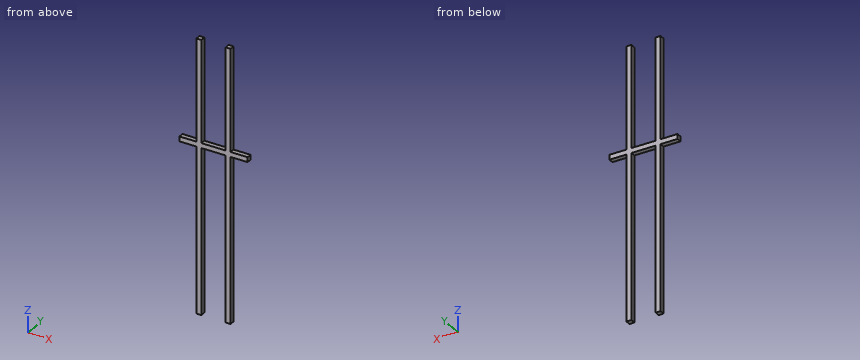
```python
from build123d import *

# Parameters (mm, degrees)
F1_DEPTH = 25.4


with BuildPart() as f1:
    # F0 (on Front) → F1 (new body)
    with BuildSketch(Plane.XZ):
        Polygon((-63.5, 546.1), (-88.9, 546.1), (-88.9, 12.7), (-177.8, 12.7), (-177.8, -12.7), (-88.9, -12.7), (-88.9, -876.3), (-63.5, -876.3), (-63.5, -12.7), (63.5, -12.7), (63.5, -876.3), (88.9, -876.3), (88.9, -12.7), (177.8, -12.7), (177.8, 12.7), (88.9, 12.7), (88.9, 546.1), (63.5, 546.1), (63.5, 12.7), (-63.5, 12.7), align=None)
    extrude(amount=-F1_DEPTH)


solid = f1.part
```
Work out the finished part from the listing and answer in its coordinate system (mm). Give positions to 0.01 mm unless a question says otherwise; leave off trailing zeros. Write each loop counter-clockwise with the first axis right and the second up, starting at its lowest first coordinate (ties: lowest second). Pieces come first, ordered by that corner, then holes. Notation, with made-up numbers: (64, -29.5) - (93, -29.5) arc R18 ccw to (93, -9.5) - close; hole circle Ø6 at (74.25, -28.75). An arc over 180 degrees is marked (long way). Use one line per item in the form item = value.
1. A cutting plane is placed at A-A (z = -176.5). Write down the section's boundary in (x, y).
Filled in:
outline = (-88.9, 0) - (-63.5, 0) - (-63.5, 25.4) - (-88.9, 25.4) - close; (63.5, 0) - (88.9, 0) - (88.9, 25.4) - (63.5, 25.4) - close
2. Each of these flat-tipped pins is pushed along its axis until it touches: pin 1 Ø1 at (x, z) = (79, 182) entering from -Y; pin 2 Ø1 at (x, y) = (59.5, 20.5) entering from -Z; pin 3 Ø12.5 at (y, z) = (13.5, 267) entering from +X; pin 4 Ø7.5 at (y, z) = (11, -463.5) entering from -X. Where does it stop, or does it pass through?
Filled in:
pin_1 = 0
pin_2 = -12.7
pin_3 = 88.9
pin_4 = -88.9
3. Consider L1, parallel to X at y = 2.75, z = -373.5; L2, parallel to Z at x = 147, y = 5.5. Determine where each line is inside the solid, lowest interval first.
Filled in:
L1 = -88.9 to -63.5, 63.5 to 88.9
L2 = -12.7 to 12.7
4. A cutting plane is placed at B-B (y = 15.75). Write down the section's boundary in (x, z).
Filled in:
outline = (-177.8, -12.7) - (-88.9, -12.7) - (-88.9, -876.3) - (-63.5, -876.3) - (-63.5, -12.7) - (63.5, -12.7) - (63.5, -876.3) - (88.9, -876.3) - (88.9, -12.7) - (177.8, -12.7) - (177.8, 12.7) - (88.9, 12.7) - (88.9, 546.1) - (63.5, 546.1) - (63.5, 12.7) - (-63.5, 12.7) - (-63.5, 546.1) - (-88.9, 546.1) - (-88.9, 12.7) - (-177.8, 12.7) - close
5. A cutting plane is placed at C-C (x = -120). Write down the section's boundary in (y, z), and give its area (3 significant figures).
Filled in:
outline = (0, -12.7) - (25.4, -12.7) - (25.4, 12.7) - (0, 12.7) - close
area = 645 mm^2
